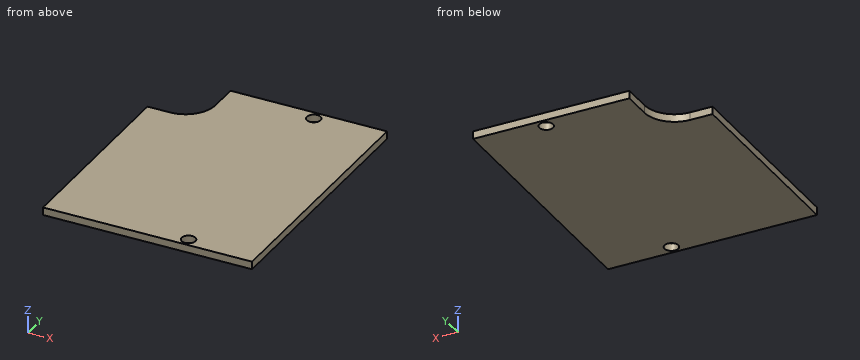
from build123d import *

# Parameters (mm, degrees)
SKETCH1_R           = 1.397
BOSS_EXTRUDE1_DEPTH = 1.5748


with BuildPart() as part:
    # Sketch1 → Boss-Extrude1 (new body)
    with BuildSketch(Plane.XY):
        with BuildLine():
            Line((0, 0), (0, 52.832))
            Line((0, 52.832), (-31.75, 52.832))
            Line((-31.75, 52.832), (-31.75, 46.99))
            ThreePointArc((-31.75, 46.99), (-33.535477062, 42.679477062), (-37.846, 40.894))
            Line((-37.846, 40.894), (-42.418, 40.894))
            Line((-42.418, 40.894), (-42.418, 0))
            Line((-42.418, 0), (0, 0))
        make_face()
        with Locations((-13.843, 50.8762)):
            Circle(SKETCH1_R, mode=Mode.SUBTRACT)
        with Locations((-13.843, 1.8542)):
            Circle(SKETCH1_R, mode=Mode.SUBTRACT)
    extrude(amount=BOSS_EXTRUDE1_DEPTH)


solid = part.part
Can you work these out from the model? Positions are in its coordinate system, mm. Round coordinates to 2 decimals unless told otherwise and drop trailing zeros. Order: outer loops, then holes, each group sorted by start corner. A loop starts at its lowest first (then second) coordinate and runs counter-clockwise, first axis right, second up. Notation, with made-up numbers: (39, -37.5) - (71, -37.5) arc R27 ccw to (71, -0.5) - close; hole circle Ø10 at (1.5, -38). An arc over 180 degrees is marked (long way). Answer in a Markdown table with one row per item.
(1) For P1, Ø4, axis at x = -24.5, y = 12.5, coming from the -Z side; P2, Ø0.8, axis at x = -40.5, z = 0.5, coming from the +Y side, each with a flat end and sliding along its axis, tell me the tip position at first contact or that it passes through.
From the geometry:
| item | result |
|---|---|
| P1 | stops at z = 0 |
| P2 | stops at y = 40.89 |
(2) Suppose I cut it at A-A, the plane z = 0.8. Please give me the cut outline in (x, y).
From the geometry:
| item | result |
|---|---|
| outline | (-42.42, 0) - (0, 0) - (0, 52.83) - (-31.75, 52.83) - (-31.75, 46.99) arc R6.1 cw to (-37.85, 40.89) - (-42.42, 40.89) - close; hole circle Ø2.79 at (-13.84, 1.85); hole circle Ø2.79 at (-13.84, 50.88) |
(3) Please list where these lines run through material, in increasing order: L1, parallel to X at y = 47.5, z = 0.3; L2, parallel to Y at x = -39.5, z = 0.8; L3, parallel to X at y = 50, z = 0.7. Write a range as from..to.
From the geometry:
| item | result |
|---|---|
| L1 | x = -31.75..0 |
| L2 | y = 0..40.89 |
| L3 | x = -31.75..-14.93, -12.75..0 |
(4) Suppose I cut it at B-B, the plane y = 48.5. Please give me the cut outline in (x, z), plus the area to 3 significant figures.
From the geometry:
| item | result |
|---|---|
| outline | (-31.75, 0) - (0, 0) - (0, 1.57) - (-31.75, 1.57) - close |
| area | 50.0 mm2 |
(5) Suppose I cut it at C-C, the plane x = -36.5. Please give me the cut outline in (y, z).
From the geometry:
| item | result |
|---|---|
| outline | (0, 0) - (41.04, 0) - (41.04, 1.57) - (0, 1.57) - close |
